from build123d import *

# Parameters (mm, degrees)
CROQUIS1_W   = 3.515255872
CROQUIS1_H   = 1.551138095
CROQUIS1_H_2 = 1.551138096


with BuildPart() as part:
    # Croquis1 → Revolución1 (revolve)
    with BuildSketch(Plane.XY, mode=Mode.PRIVATE) as revoluci_n1_sk:
        with BuildLine():
            ThreePointArc((3.25, 12.5), (4.75, 11), (3.25, 9.5))
            Line((3.25, 9.5), (3.25, -7.5))
            Line((3.25, -7.5), (6.75, -7.5))
            Line((6.75, -7.5), (7.75, -8.5))
            Line((7.75, -8.5), (7.75, -12.5))
            Line((7.75, -12.5), (1.25, -12.5))
            Line((1.25, -12.5), (1.25, 12.5))
            Line((1.25, 12.5), (3.25, 12.5))
        make_face()
        with Locations((3.007627936, -13.275569047)):
            Rectangle(CROQUIS1_W, CROQUIS1_H)
        with Locations((3.007627936, -14.826707143)):
            Rectangle(CROQUIS1_W, CROQUIS1_H_2)
        with BuildLine():
            Line((7.75, -15.602276191), (4.765255872, -15.602276191))
            Line((4.765255872, -15.602276191), (1.25, -15.602276191))
            Line((1.25, -15.602276191), (1.25, -40.602276191))
            Line((1.25, -40.602276191), (3.25, -40.602276191))
            ThreePointArc((3.25, -40.602276191), (4.75, -39.102276191), (3.25, -37.602276191))
            Line((3.25, -37.602276191), (3.25, -20.602276191))
            Line((3.25, -20.602276191), (6.75, -20.602276191))
            Line((6.75, -20.602276191), (7.75, -19.602276191))
            Line((7.75, -19.602276191), (7.75, -15.602276191))
        make_face()
    revolve(revoluci_n1_sk.sketch.rotate(Axis((-7.75, -7.5, 0), (0, 1, 0)), 90), axis=Axis((-7.75, -7.5, 0), (0, 1, 0)))


solid = part.part
CAD build for the part. Positions are in the model's coordinates, mm. A direction names the side the tool comes from. Round coordinates to 2 decimals unless told otherwise and drop trailing zeros. Write each loop counter-clockwise with the first axis right and the second up, starting at its lowest first coordinate (ties: lowest second). Pieces come first, ordered by that corner, then holes. Notation, with made-up numbers: (-8, -29) -> (33, -29) arc R17 ccw to (33, -4) -> close; hole circle Ø1 at (14.25, 27). An arc over 180 degrees is marked (long way). Answer as a JSON object with one key per item and string values.
(1) Pin check, flat tips, straight feed: P1, Ø8, axis at x = -18.5, y = 2.5, coming from the +Z side; P2, Ø3, axis at x = -17.5, z = -9.5, coming from the -Y side; P3, Ø6, axis at x = 1.5, y = -34.5, coming from the -Z side; P4, Ø9.5, axis at x = -10, z = 2, coming from the +Y side. Stop position of each tip, or through.
Reported:
{"P1": "stops at z = 8.69", "P2": "stops at y = -40.11", "P3": "stops at z = -9.05", "P4": "passes through"}
(2) Probe probe 1 along Y at (x, z) = (-10, -14); probe 2 along X at (y, z) = (-23, 0); probe 3 along Y at (x, z) = (2, -7). List the from-to ranges inside material, lowest first. Write a range as [from, to].
Reported:
{"probe 1": "y = [-20.6, -15.6], [-12.5, -7.5]", "probe 2": "x = [-18.75, -16.75], [1.25, 3.25]", "probe 3": "y = [-40.22, -37.99], [-20.6, -7.5], [9.88, 12.12]"}
(3) Band-saw the part on C-C, the plane y = -23.5. List the corners of the cut face in (x, z).
Reported:
{"outline": "circle Ø22 at (-7.75, 0); hole circle Ø18 at (-7.75, 0)"}
(4) Which spindle directions (+Z, -Z, +X, -X, +Y, -Y) get a long thin tool onto all of the face, cutting with end or side? Do faces 4 (the face through (2.99, -28.98, 2.38)), 5 (the face through (7.38, -10.53, 3.36)). Say none if no direction does.
Reported:
{"face 4": "none", "face 5": "+Y, -Y"}
(5) Two-plate mould, pull along X, no slides. Class faces 1 (the face through (1.036, -14.423, 1.951)), 2 (the face through (-8, -8, 15)), 3 (the face through (-19, -20.602, -2)): +X half, -X half, draft (parallel to the pull), parting line (faces both ways), or undercut.
Reported:
{"face 1": "undercut", "face 2": "parting line", "face 3": "draft"}
